from build123d import *

# Parameters (mm, degrees)
F0_W     = 60
F0_H     = 50
F1_DEPTH = 20
F2_DEPTH = 50
F3_R     = 5


with BuildPart() as f1:
    # F0 (on Top) → F1 (new body)
    with BuildSketch(Plane.XY):
        with Locations((-30, 32.220189)):
            Rectangle(F0_W, F0_H)
    extrude(amount=F1_DEPTH)

    # F0 (on Top) → F2 (join)
    with BuildSketch(Plane.XY):
        Polygon((0, 57.220189), (0, 7.220189), (20, 7.220189), (20, 17.220189), (12, 17.220189), (12, 47.220189), (20, 47.220189), (20, 57.220189), align=None)
    extrude(amount=F2_DEPTH)

    # F3
    f3_edges = [f1.edges().sort_by_distance(p)[0] for p in [
        (0, 32.220189, 50),
        (-60, 32.220189, 20),
    ]]
    fillet(f3_edges, radius=F3_R)


solid = f1.part
Input: part model. Units: mm. Frame: model coordinates. A direction names the side the tool comes from. Give positions to 0.01 mm unless a question says otherwise; leave off trailing zeros. Order: outer loops, then holes, each group sorted by start corner. A loop starts at its lowest first (then second) coordinate and runs counter-clockwise, first axis right, second up. Notation, with made-up numbers: (-28.5, 48.5) - (26.5, 48.5) arc R19 ccw to (26.5, 67.5) - close; hole circle Ø7 at (-36.5, 49.25). An arc over 180 degrees is marked (long way). Answer as a JSON object with one key per item and string values. Group by question number.
Q1. Set-up query: faces 1 (the face through (16, 47.22, 25)), 2 (the face through (0, 33, 32)), 3 (the face through (20, 12, 25)). Return all of +Z, -Z, +X, -X, +Y, -Y with unobstructed straight access to the full face (end or side cutting, diameter ignored); none if empty.
Q2. Line query: probe 1 along Z at (x, y) = (-46, 51); probe 2 along X at (y, z) = (38, 12); probe 3 along X at (y, z) = (19, 32.5). Output: solid intervals per line, ascending.
Q3. Cut plane A-A, the plane y = 51.5. Output: boundary loops of the cut face in (x, z).
Q4. Cut plane B-B, the plane z = 34.5. Output: boundary loops of the cut face in (x, y).
Q5. First-contact query: pin 1 Ø20 at (y, z) = (40.5, 27.5) entering from -X; pin 2 Ø24 at (y, z) = (32.5, 34) entering from +X; pin 3 Ø10 at (x, y) = (-29.5, 21.5) entering from +Z. Flat tips, straight axial feed; report the tip coordinate or a pass-through.
Q6. Cut plane C-C, the plane x = -9. Output: boundary loops of the cut face in (y, z), then the cut area to 3 significant figures.
Q7. Mould query, pull axis Y, two halves, no side actions, for faces 4 (the face through (16, 17.22, 25)), 5 (the face through (-28, 33, 20)), 6 (the face through (-11, 57.22, 14)). Classes: pulls with the +Y half, pulls with the -Y half, needs draft (parallel to the pull), parting line crosses it, or undercut.
Results:
{
 "1": {"face 1": "+Z, -Z, +X", "face 2": "+Z, -X, +Y, -Y", "face 3": "+Z, -Z, +X, +Y, -Y"},
 "2": {"probe 1": "0 to 20", "probe 2": "-60 to 12", "probe 3": "0 to 12"},
 "3": {"outline": "(-60, 0) - (20, 0) - (20, 50) - (5, 50) arc R5 ccw to (0, 45) - (0, 20) - (-55, 20) arc R5 ccw to (-60, 15) - close"},
 "4": {"outline": "(0, 7.22) - (20, 7.22) - (20, 17.22) - (12, 17.22) - (12, 47.22) - (20, 47.22) - (20, 57.22) - (0, 57.22) - close"},
 "5": {"pin 1": "x = -59.33", "pin 2": "x = 12", "pin 3": "z = 20"},
 "6": {"outline": "(7.22, 0) - (57.22, 0) - (57.22, 20) - (7.22, 20) - close", "area": "1,000 mm^2"},
 "7": {"face 4": "undercut", "face 5": "needs draft", "face 6": "pulls with the +Y half"}
}
